Part print with two shaded views. Sizes in mm from the minimum x, y, z corner. Round coordinates to 2 decimals unless told otherwise and drop trailing zeros. Order: outer loops, then holes, each group sorted by start corner. A loop starts at its lowest first (then second) coordinate and runs counter-clockwise, first axis right, second up. Notation, with made-up numbers: (-14.75, 4.5) -> (27.25, 4.5) arc R15 ccw to (27.25, 20.5) -> close; hole circle Ø9 at (53.25, -4). An arc over 180 degrees is marked (long way). Put each result on its own line as item: value. Start each with the question number.
Q1. Cut at C-C, the plane x = 170.7. List the corners of the cut face in (y, z), and give its area (3 significant figures).
Q2. Flat gauge pin, fed straight in: P1, Ø1.9, axis at x = 62.7, z = 41, coming from the -Y side. Where does the tip first touch, or does it go through?
Q3. Cut at B-B, the plane y = 3.4. State how many separate pieces and enclosed holes the cut face has, and give its area (3 significant figures).
Q4. Probe L1, parallel to X at y = 1.05, z = 35; L2, parallel to Z at x = 62.7, y = 1; L3, parallel to X at y = 3.2, z = 4. List the from-to ranges inside material, lowest first.
Q5. Cut at A-A, the plane z = 53. List the corners of the cut face in (x, y).
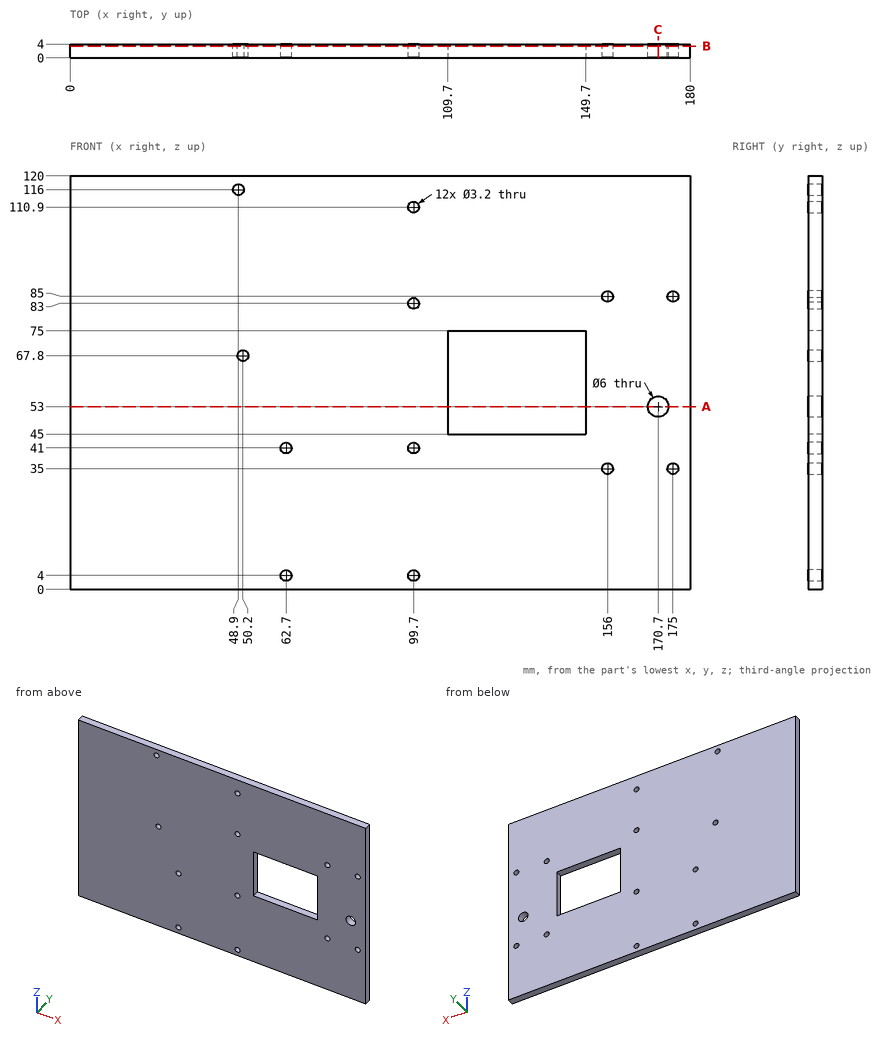
Ans:
1. outline: (0, 0) -> (4, 0) -> (4, 50) -> (0, 50) -> close; (0, 56) -> (4, 56) -> (4, 120) -> (0, 120) -> close
1. area: 456 mm^2
2. P1: passes through
3. separate pieces: 1
3. enclosed holes: 14
3. area: 20,300 mm^2
4. L1: x = 0 to 154.4, 157.6 to 173.4, 176.6 to 180
4. L2: z = 0 to 2.4, 5.6 to 39.4, 42.6 to 120
4. L3: x = 0 to 61.1, 64.3 to 98.1, 101.3 to 180
5. outline: (0, 0) -> (109.7, 0) -> (109.7, 4) -> (0, 4) -> close; (149.7, 0) -> (167.7, 0) -> (167.7, 4) -> (149.7, 4) -> close; (173.7, 0) -> (180, 0) -> (180, 4) -> (173.7, 4) -> close
